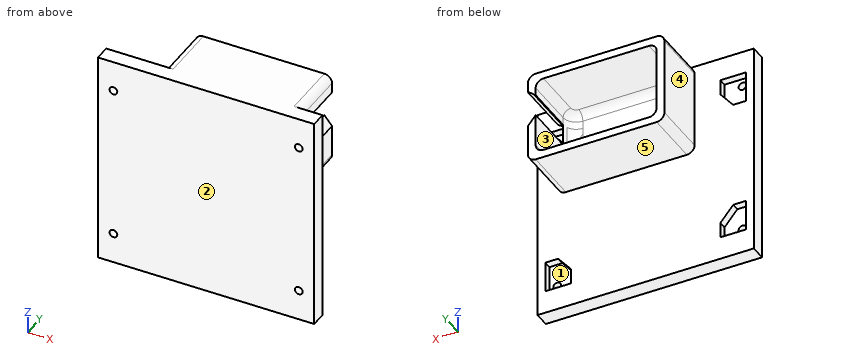
from build123d import *

# Parameters (mm, degrees)
SKETCH1_W               = 84
SKETCH1_H               = 84
BOSS_EXTRUDE1_DEPTH     = 6
SKETCH2_R               = 1.5
CUT_EXTRUDE1_DEPTH      = 119.94536561
SKETCH4_R               = 1.5
CUT_EXTRUDE4_DEPTH      = 3
MIRROR3_COPY_1_SKETCH_R = 1.5
MIRROR3_COPY_1_DEPTH    = 3
SKETCH5_W               = 53
SKETCH5_H               = 36
BOSS_EXTRUDE2_DEPTH     = 22
SKETCH6_W               = 47
SKETCH6_H               = 30
CUT_EXTRUDE5_DEPTH      = 25
FILLET1_R               = 3
FILLET2_R               = 5
BOSS_EXTRUDE3_START     = -17.4
BOSS_EXTRUDE3_DEPTH     = 8.4
CUT_EXTRUDE14_START     = -22
CUT_EXTRUDE14_DEPTH     = 22
CUT_EXTRUDE15_DEPTH     = 122.396046085


# Read off the part's stored shape, not the designer's step: Boss-Extrude3
with BuildPart() as part:
    # Sketch1 → Boss-Extrude1 (new body)
    with BuildSketch(Plane(origin=(0, 0, 0), x_dir=(1, 0, 0), z_dir=(0, 1, 0))):
        with Locations((42, 42)):
            Rectangle(SKETCH1_W, SKETCH1_H)
    extrude(amount=BOSS_EXTRUDE1_DEPTH)

    # Sketch2 → Cut-Extrude1 (cut, through all)
    with BuildSketch(Plane(origin=(0, 6, 0), x_dir=(1, 0, 0), z_dir=(0, 1, 0))):
        with Locations(Location((6, 72, 0), (0, 0, 270))):
            Circle(SKETCH2_R)
        with Locations(Location((6, 12, 0), (0, 0, 270))):
            Circle(SKETCH2_R)
        with Locations(Location((78, 12, 0), (0, 0, 270))):
            Circle(SKETCH2_R)
        with Locations(Location((78, 72, 0), (0, 0, 270))):
            Circle(SKETCH2_R)
    extrude(amount=-CUT_EXTRUDE1_DEPTH, mode=Mode.SUBTRACT)

    # Sketch4 → Cut-Extrude4 (cut)
    with BuildSketch(Plane(origin=(0, 6, 0), x_dir=(1, 0, 0), z_dir=(0, 1, 0))):
        Polygon((13, 15), (13, 9), (3, 9), (3, 21), (8, 21), align=None)
        with Locations(Location((6, 12, 0), (0, 0, 270))):
            Circle(SKETCH4_R, mode=Mode.SUBTRACT)
    cut_extrude4 = extrude(amount=-CUT_EXTRUDE4_DEPTH, mode=Mode.SUBTRACT)

    # Mirror2: Cut-Extrude4 across plane
    add(cut_extrude4.mirror(Plane.XY.offset(-42)), mode=Mode.SUBTRACT)

    # Mirror3: Cut-Extrude4 across plane
    add(cut_extrude4.mirror(Plane.ZY.offset(-42)), mode=Mode.SUBTRACT)

    # Mirror3 copy 1 sketch → Mirror3 copy 1 (cut)
    with BuildSketch(Plane(origin=(84, 6, -84), x_dir=(-1, 0, 0), z_dir=(0, 1, 0))):
        Polygon((13, 15), (13, 9), (3, 9), (3, 21), (8, 21), align=None)
        with Locations(Location((6, 12, 0), (0, 0, 270))):
            Circle(MIRROR3_COPY_1_SKETCH_R, mode=Mode.SUBTRACT)
    extrude(amount=-MIRROR3_COPY_1_DEPTH, mode=Mode.SUBTRACT)

    # Sketch5 → Boss-Extrude2 (add)
    with BuildSketch(Plane(origin=(0, 6, 0), x_dir=(1, 0, 0), z_dir=(0, 1, 0))):
        with Locations((49.5, 18)):
            Rectangle(SKETCH5_W, SKETCH5_H)
    extrude(amount=BOSS_EXTRUDE2_DEPTH)

    # Sketch6 → Cut-Extrude5 (cut)
    with BuildSketch(Plane(origin=(0, 28, 0), x_dir=(1, 0, 0), z_dir=(0, 1, 0))):
        with Locations((49.5, 18)):
            Rectangle(SKETCH6_W, SKETCH6_H)
    extrude(amount=-CUT_EXTRUDE5_DEPTH, mode=Mode.SUBTRACT)

    # Fillet1
    fillet1_edges = [part.edges().sort_by_distance(p)[0] for p in [
        (76, 17, -36),
        (23, 17, -36),
        (23, 17, 0),
        (76, 17, 0),
        (73, 15.5, -33),
        (49.5, 3, -3),
        (73, 15.5, -3),
        (26, 15.5, -3),
        (49.5, 3, -33),
        (26, 15.5, -33),
    ]]
    fillet(fillet1_edges, radius=FILLET1_R)

    # Fillet2
    # the kernel refuses this fillet: 5 mm, written as the material it adds along each edge
    with BuildSketch(Plane(origin=(31, 8, -3), x_dir=(-1, 0, 0), z_dir=(0, 1, 0))) as fillet2_piece_1:
        with BuildLine():
            CenterArc((2, -3), 3, 0, 90)
            Line((5, -3), (5, 0))
            Line((5, 0), (2, 0))
        make_face()
    revolve(axis=Axis((31, 8, -3), (0, 0, 1)), revolution_arc=90)
    with BuildSketch(Plane(origin=(31, 8, -33), x_dir=(0, -1, 0), z_dir=(1, 0, 0))) as fillet2_piece_2:
        with BuildLine():
            CenterArc((2, -3), 3, 0, 90)
            Line((5, -3), (5, 0))
            Line((5, 0), (2, 0))
        make_face()
    revolve(axis=Axis((31, 8, -33), (0, 0, -1)), revolution_arc=90)
    with BuildSketch(Plane(origin=(68, 8, -3), x_dir=(0, -1, 0), z_dir=(-1, 0, 0))) as fillet2_piece_3:
        with BuildLine():
            CenterArc((2, -3), 3, 0, 90)
            Line((5, -3), (5, 0))
            Line((5, 0), (2, 0))
        make_face()
    revolve(axis=Axis((68, 8, -3), (0, 0, 1)), revolution_arc=90)
    with BuildSketch(Plane(origin=(73, 3, -4.9), x_dir=(-1, 0, 0), z_dir=(0, 0, -1))) as fillet2_piece_4_section:
        with BuildLine():
            CenterArc((FILLET2_R, FILLET2_R), FILLET2_R, 180, 90)
            Line((0, FILLET2_R), (0, 0))
            Line((0, 0), (FILLET2_R, 0))
        make_face()
    fillet2_piece_4 = extrude(amount=37.6, mode=Mode.PRIVATE)
    fillet2_piece_4 = split(fillet2_piece_4, bisect_by=Plane(origin=(71.840443932, 4.051726495, -9), z_dir=(0, 0, 1)), keep=Keep.TOP, mode=Mode.PRIVATE)
    add(fillet2_piece_4)
    with BuildSketch(Plane(origin=(73, 3, -4.9), x_dir=(-1, 0, 0), z_dir=(0, 0, -1))) as fillet2_piece_5_section:
        with BuildLine():
            CenterArc((FILLET2_R, FILLET2_R), FILLET2_R, 180, 90)
            Line((0, FILLET2_R), (0, 0))
            Line((0, 0), (FILLET2_R, 0))
        make_face()
    fillet2_piece_5 = extrude(amount=37.6, mode=Mode.PRIVATE)
    fillet2_piece_5 = split(fillet2_piece_5, bisect_by=Plane(origin=(72.877053979, 6.49875804, -36), z_dir=(0, 0, 1)), keep=Keep.TOP, mode=Mode.PRIVATE)
    fillet2_piece_5 = split(fillet2_piece_5, bisect_by=Plane(origin=(72.877053979, 6, -13.126232387), z_dir=(0, 1, 0)), keep=Keep.TOP, mode=Mode.PRIVATE)
    add(fillet2_piece_5)
    with BuildSketch(Plane(origin=(73, 3, -4.9), x_dir=(-1, 0, 0), z_dir=(0, 0, -1))) as fillet2_piece_6_section:
        with BuildLine():
            CenterArc((FILLET2_R, FILLET2_R), FILLET2_R, 180, 90)
            Line((0, FILLET2_R), (0, 0))
            Line((0, 0), (FILLET2_R, 0))
        make_face()
    fillet2_piece_6 = extrude(amount=37.6, mode=Mode.PRIVATE)
    fillet2_piece_6 = split(fillet2_piece_6, bisect_by=Plane(origin=(74.593810092, 3.935909556, -19.312572111), z_dir=(-0.7682212795973755, 0, -0.6401843996644804)), keep=Keep.TOP, mode=Mode.PRIVATE)
    fillet2_piece_6 = split(fillet2_piece_6, bisect_by=Plane(origin=(71.754876355, 6, -21.678350226), z_dir=(0, -1, 0)), keep=Keep.TOP, mode=Mode.PRIVATE)
    add(fillet2_piece_6)
    with BuildSketch(Plane(origin=(73, 3, -3), x_dir=(-1, 0, 0), z_dir=(0, 0, -1))) as fillet2_piece_7:
        with BuildLine():
            CenterArc((FILLET2_R, FILLET2_R), FILLET2_R, 180, 90)
            Line((0, FILLET2_R), (0, 0))
            Line((0, 0), (FILLET2_R, 0))
        make_face()
    extrude(amount=6)
    with BuildSketch(Plane(origin=(73, 3, -3), x_dir=(-1, 0, 0), z_dir=(0, 0, -1))) as fillet2_piece_8_section:
        with BuildLine():
            CenterArc((FILLET2_R, FILLET2_R), FILLET2_R, 180, 90)
            Line((0, FILLET2_R), (0, 0))
            Line((0, 0), (FILLET2_R, 0))
        make_face()
    fillet2_piece_8 = extrude(amount=18.5, mode=Mode.PRIVATE)
    fillet2_piece_8 = split(fillet2_piece_8, bisect_by=Plane(origin=(72.877053979, 6, -13.126232386), z_dir=(0, 1, 0)), keep=Keep.TOP, mode=Mode.PRIVATE)
    add(fillet2_piece_8)
    with BuildSketch(Plane(origin=(73, 3, -3), x_dir=(-1, 0, 0), z_dir=(0, 0, -1))) as fillet2_piece_9_section:
        with BuildLine():
            CenterArc((FILLET2_R, FILLET2_R), FILLET2_R, 180, 90)
            Line((0, FILLET2_R), (0, 0))
            Line((0, 0), (FILLET2_R, 0))
        make_face()
    fillet2_piece_9 = extrude(amount=18.5, mode=Mode.PRIVATE)
    fillet2_piece_9 = split(fillet2_piece_9, bisect_by=Plane(origin=(73.049643728, 3.899661729, -17.459572473), z_dir=(-0.7682212795973755, 0, -0.6401843996644804)), keep=Keep.TOP, mode=Mode.PRIVATE)
    add(fillet2_piece_9)
    with BuildSketch(Plane(origin=(26, 3, -33), x_dir=(1, 0, 0), z_dir=(0, 0, 1))) as fillet2_piece_10:
        with BuildLine():
            CenterArc((FILLET2_R, FILLET2_R), FILLET2_R, 180, 90)
            Line((0, FILLET2_R), (0, 0))
            Line((0, 0), (FILLET2_R, 0))
        make_face()
    extrude(amount=30)

    # Boss-Extrude3 outline → Boss-Extrude3 (add)
    with BuildSketch(Plane.XY.offset(BOSS_EXTRUDE3_START)):
        with BuildLine():
            Line((73, 6), (72.582575695, 6))
            ThreePointArc((72.582575695, 6), (70.738612788, 3.816699867), (68, 3))
            Line((68, 3), (73, 3))
            Line((73, 3), (73, 6))
        make_face()
    extrude(amount=BOSS_EXTRUDE3_DEPTH)

    # Sketch8 → Cut-Extrude14 (cut)
    with BuildSketch(Plane(origin=(0, 28, 0), x_dir=(1, 0, 0), z_dir=(0, 1, 0)).offset(CUT_EXTRUDE14_START)):
        with BuildLine():
            Line((76, 9), (76, 17.123475383))
            ThreePointArc((76, 17.123475383), (74.22437799, 15.99933475), (73, 14.291287847))
            Line((73, 14.291287847), (73, 9.708712153))
            ThreePointArc((73, 9.708712153), (73.182064882, 9.347171095), (73.390227771, 9))
            Line((73.390227771, 9), (76, 9))
        make_face()
        with BuildLine():
            Line((76, 6.876524617), (76, 9))
            Line((76, 9), (73.390227771, 9))
            ThreePointArc((73.390227771, 9), (74.528752508, 7.733802531), (76, 6.876524617))
        make_face()
    extrude(amount=CUT_EXTRUDE14_DEPTH, mode=Mode.SUBTRACT)

    # Sketch13 → Cut-Extrude15 (cut, through all)
    with BuildSketch(Plane(origin=(0, 3, 0), x_dir=(1, 0, 0), z_dir=(0, 1, 0))):
        Polygon((73, 17.4), (73, 9), (81, 9), (81, 21), (76, 21), align=None)
    extrude(amount=CUT_EXTRUDE15_DEPTH, mode=Mode.SUBTRACT)


solid = part.part
Verification items for the finished model (mm, model axes). Face numbers are marked on the shaded views. A direction names the side the tool comes from. Give positions to 0.01 mm unless a question says otherwise; leave off trailing zeros. Loops run counter-clockwise (first coordinate to the right, second up) from the corner with the lowest first, then second, coordinate; pieces in that order, holes last.
1) Sectioned sample at C-C, the plane y = 20. Enter the section's corners in (x, z).
2) Sectioned sample at B-B, the plane z = -72. Enter the section's corners in (x, y), then the cut area to 3 significant figures.
3) Depth check by flat-ended pin: pin 1 Ø3 at (x, z) = (6, -66) entering from +Y; pin 2 Ø14 at (y, z) = (17, -25) entering from -X; pin 3 Ø6.5 at (x, y) = (55.5, 15.5) entering from -Z. Enter the tip coordinate at first touch or a pass-through.
4) Sectioned sample at D-D, the plane x = 53. Enter the section's corners in (y, z), then the cut area to 3 significant figures.
5) Draft check along Z on the marked faces 3, 4 and 5. Enter one of: pulls with the +Z half, pulls with the -Z half, needs draft (parallel to the pull), parting line crosses it, or undercut.
6) Thickness scan on line 1 along X through (y, z) = (2.1, -12); line 2 along Z through (x, y) = (78, 2.15); line 3 along Z through (x, y) = (56, 23.5). Record the ranges inside material, lowest first.
7) Sectioned sample at A-A, the plane x = 6. Enter the section's corners in (y, z).
8) Set-up check for the marked faces 1 and 2: record each of +Z, -Z, +X, -X, +Y, -Y from which the full face is reachable in a straight line by a thin tool's end or side.
Answers:
1. outline: (23, -33) arc R3 ccw to (26, -36) - (73, -36) arc R3 ccw to (76, -33) - (76, -21) - (73, -17.4) - (73, -30) arc R3 cw to (70, -33) - (29, -33) arc R3 cw to (26, -30) - (26, -6) arc R3 cw to (29, -3) - (70, -3) arc R3 cw to (73, -6) - (73, -9) - (73.39, -9) arc R5.5 cw to (76, -6.88) - (76, -3) arc R3 ccw to (73, 0) - (26, 0) arc R3 ccw to (23, -3) - close
2. outline: (0, 0) - (4.5, 0) - (4.5, 3) - (3, 3) - (3, 6) - (0, 6) - close; (7.5, 0) - (76.5, 0) - (76.5, 3) - (71, 3) - (71, 6) - (13, 6) - (13, 3) - (7.5, 3) - close; (79.5, 0) - (84, 0) - (84, 6) - (81, 6) - (81, 3) - (79.5, 3) - close
2. area: 426 mm2
3. pin 1: stops at y = 3
3. pin 2: stops at x = 23
3. pin 3: stops at z = -36
4. outline: (0, -84) - (6, -84) - (6, -36) - (28, -36) - (28, -33) - (6, -33) arc R3 cw to (3, -30) - (3, -6) arc R3 cw to (6, -3) - (28, -3) - (28, 0) - (0, 0) - close
4. area: 550 mm2
5. face 3: undercut
5. face 4: needs draft
5. face 5: pulls with the -Z half
6. line 1: x = 0 to 4.5, 7.5 to 76.5, 79.5 to 84
6. line 2: z = -84 to -73.5, -70.5 to -13.5, -10.5 to 0
6. line 3: z = -36 to -33, -3 to 0
7. outline: (0, -84) - (6, -84) - (6, -75) - (3, -75) - (3, -73.5) - (0, -73.5) - close; (0, -70.5) - (3, -70.5) - (3, -63) - (6, -63) - (6, -21) - (3, -21) - (3, -13.5) - (0, -13.5) - close; (0, -10.5) - (3, -10.5) - (3, -9) - (6, -9) - (6, 0) - (0, 0) - close
8. face 1: +Y
8. face 2: +Z, -Z, +X, -X, -Y
